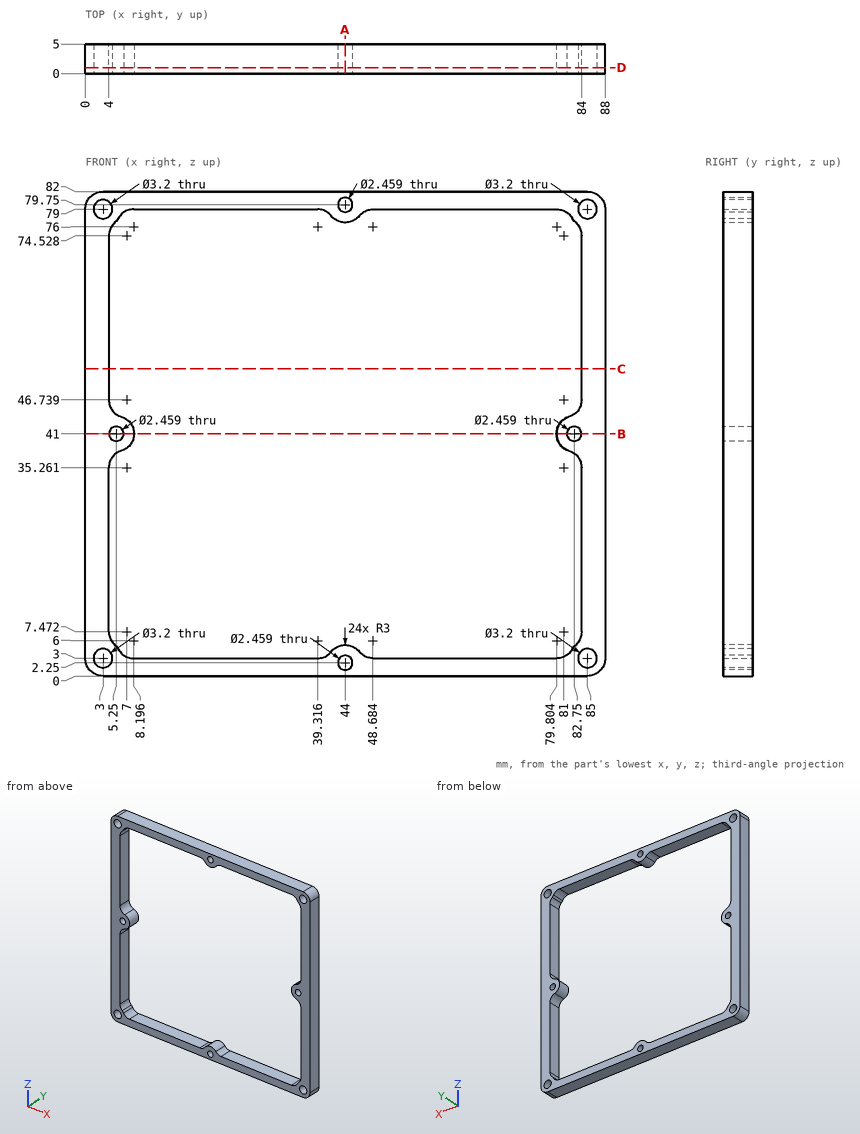
Could you check a few things on this drawing? It's one solid part, dimensions in mm from its lowest x, y, z. Round coordinates to 2 decimals unless told otherwise and drop trailing zeros. Order: outer loops, then holes, each group sorted by start corner. A loop starts at its lowest first (then second) coordinate and runs counter-clockwise, first axis right, second up. Notation, with made-up numbers: M 39,71 L 51,71 A19 cw 51,75 Z; hole C -2,-33 d10. An arc over 180 degrees is marked long. One line per question, with ' | ' between items. Start each with the question number.
(1) Suppose I cut it at B-B on z = 41. List the corners of the cut face in (x, y) for me, then the cut area to 3 significant figures.
(2) Suppose I cut it at A-A on x = 44. List the corners of the cut face in (y, z) for me.
(3) Please list where these lines run through material, in increasing order: line 1 along Z through (x, y) = (85, 3.7); line 2 along X through (y, z) = (4.35, 15); line 3 along X through (y, z) = (2.05, 41).
(4) For P1, Ø3, axis at x = 3, z = 3, coming from the +Y side; P2, Ø3, axis at x = 44, z = 79.75, coming from the -Y side, each with a flat end and sliding along its axis, tell me the tip position at first contact or that it passes through.
(5) Suppose I cut it at C-C on z = 52. List the corners of the cut face in (x, y) for me.
(6) Suppose I cut it at D-D on y = 1. Count the separate pieces of the cut face and the enclosed holes in it, then the cut area to 3 significant figures.
Geometry results:
1) outline: M 0,0 L 4.02,0 L 4.02,5 L 0,5 Z; M 6.48,0 L 8.25,0 L 8.25,5 L 6.48,5 Z; M 79.75,0 L 81.52,0 L 81.52,5 L 79.75,5 Z; M 83.98,0 L 88,0 L 88,5 L 83.98,5 Z | area: 57.9 mm²
2) outline: M 0,0 L 5,0 L 5,1.02 L 0,1.02 Z; M 0,3.48 L 5,3.48 L 5,5.25 L 0,5.25 Z; M 0,76.75 L 5,76.75 L 5,78.52 L 0,78.52 Z; M 0,80.98 L 5,80.98 L 5,82 L 0,82 Z
3) line 1: 0 to 1.4, 4.6 to 77.4, 80.6 to 82 | line 2: 0 to 4, 84 to 88 | line 3: 0 to 4.02, 6.48 to 8.25, 79.75 to 81.52, 83.98 to 88
4) P1: through | P2: y = 0
5) outline: M 0,0 L 4,0 L 4,5 L 0,5 Z; M 84,0 L 88,0 L 88,5 L 84,5 Z
6) separate pieces: 1 | enclosed holes: 9 | area: 1,170 mm²
